```python
from build123d import *

# Parameters (mm, degrees)
SKETCH1_W                    = 91
SKETCH1_H                    = 32
BASE_FLANGE1_DEPTH           = 2
EDGE_FLANGE1_STRIP_W         = 14
EDGE_FLANGE1_STRIP_H         = 2
EDGE_FLANGE1_STRIP_CUT_DEPTH = 32
EDGE_FLANGE1_DEPTH           = 32
EDGE_FLANGE2_STRIP_W         = 14
EDGE_FLANGE2_STRIP_H         = 2
EDGE_FLANGE2_STRIP_CUT_DEPTH = 32
EDGE_FLANGE2_DEPTH           = 32
FILLET1_R                    = 3
EDGE_FLANGE3_DEPTH           = 29
EDGE_FLANGE3_START           = 2
EDGE_FLANGE3_FLAT_DEPTH      = 2
EDGE_FLANGE4_DEPTH           = 20
EDGE_FLANGE4_START           = 2
EDGE_FLANGE4_PROFILE_R       = 4
EDGE_FLANGE4_FLAT_DEPTH      = 2
SKETCH18_R                   = 6.5
CUT_EXTRUDE1_DEPTH           = 10
EDGE_FLANGE5_DEPTH           = 6
EDGE_FLANGE5_START           = 2
EDGE_FLANGE5_FLAT_DEPTH      = 2
EDGE_FLANGE6_STRIP_W         = 14
EDGE_FLANGE6_STRIP_H         = 2
EDGE_FLANGE6_STRIP_CUT_DEPTH = 32
EDGE_FLANGE6_DEPTH           = 32
EDGE_FLANGE7_STRIP_W         = 14
EDGE_FLANGE7_STRIP_H         = 2
EDGE_FLANGE7_STRIP_CUT_DEPTH = 32
EDGE_FLANGE7_DEPTH           = 32
EDGE_FLANGE7_FLAT_DEPTH      = 2
CUT_EXTRUDE2_DEPTH           = 10


# Sheet-metal steps are written as plain solids
with BuildPart() as part:
    # Sketch1 → Base-Flange1 (new body)
    with BuildSketch(Plane(origin=(0, 0, 0), x_dir=(0, 1, 0), z_dir=(0, 0, 1))):
        with Locations((-3.5, -1)):
            Rectangle(SKETCH1_W, SKETCH1_H)
    extrude(amount=BASE_FLANGE1_DEPTH)

    # Edge-Flange1 strip (across the edge) → Edge-Flange1 strip cut (cut)
    with BuildSketch(Plane(origin=(-15, -49, 2), x_dir=(0, 1, 0), z_dir=(1, 0, 0))):
        with Locations((-2, -1)):
            Rectangle(EDGE_FLANGE1_STRIP_W, EDGE_FLANGE1_STRIP_H)
    extrude(amount=EDGE_FLANGE1_STRIP_CUT_DEPTH, mode=Mode.SUBTRACT)

    # Edge-Flange1 section (across the edge) → Edge-Flange1 (add)
    with BuildSketch(Plane(origin=(-15, -49, 2), x_dir=(0, 1, 0), z_dir=(1, 0, 0))):
        with BuildLine():
            Line((0, 3), (0, 41))
            Line((0, 41), (2, 41))
            Line((2, 41), (2, 3))
            ThreePointArc((2, 3), (2.878679656, 0.878679656), (5, 0))
            Line((5, 0), (5, -2))
            ThreePointArc((5, -2), (1.464466094, -0.535533906), (0, 3))
        make_face()
    extrude(amount=EDGE_FLANGE1_DEPTH)

    # Edge-Flange2 strip (across the edge) → Edge-Flange2 strip cut (cut)
    with BuildSketch(Plane(origin=(17, -49, 43), x_dir=(0, 0, -1), z_dir=(-1, 0, 0))):
        with Locations((-2, -1)):
            Rectangle(EDGE_FLANGE2_STRIP_W, EDGE_FLANGE2_STRIP_H)
    extrude(amount=EDGE_FLANGE2_STRIP_CUT_DEPTH, mode=Mode.SUBTRACT)

    # Edge-Flange2 section (across the edge) → Edge-Flange2 (add)
    with BuildSketch(Plane(origin=(17, -49, 43), x_dir=(0, 0, -1), z_dir=(-1, 0, 0))):
        with BuildLine():
            Line((0, 3), (0, 19))
            Line((0, 19), (2, 19))
            Line((2, 19), (2, 3))
            ThreePointArc((2, 3), (2.878679656, 0.878679656), (5, 0))
            Line((5, 0), (5, -2))
            ThreePointArc((5, -2), (1.464466094, -0.535533906), (0, 3))
        make_face()
    extrude(amount=EDGE_FLANGE2_DEPTH)

    # Fillet1
    fillet1_edges = [part.edges().sort_by_distance(p)[0] for p in [
        (17, -68, 42),
        (-15, -68, 42),
    ]]
    fillet(fillet1_edges, radius=FILLET1_R)

    # Edge-Flange3 bend section (across the edge) → Edge-Flange3 (add)
    with BuildSketch(Plane(origin=(20, -33, 2), x_dir=(-1, 0, 0), z_dir=(0, 1, 0))):
        with BuildLine():
            Line((-2, 3), (0, 3))
            ThreePointArc((0, 3), (0.878679656, 0.878679656), (3, 0))
            Line((3, 0), (3, -2))
            ThreePointArc((3, -2), (-0.535533906, -0.535533906), (-2, 3))
        make_face()
    extrude(amount=EDGE_FLANGE3_DEPTH)

    # Edge-Flange3 profile (on flange) → Edge-Flange3 flat (add)
    with BuildSketch(Plane(origin=(20, 0, 2), x_dir=(0, 1, 0), z_dir=(1, 0, 0)).offset(EDGE_FLANGE3_START)):
        with BuildLine():
            Line((-33, 41), (-33, 3))
            Line((-33, 3), (-4, 3))
            Line((-4, 3), (-4, 7))
            Line((-4, 7), (7.090242207, 7))
            ThreePointArc((7.090242207, 7), (9, 8.406009114), (8.22462093, 10.647174828))
            Line((8.22462093, 10.647174828), (-1, 17))
            Line((-1, 17), (-13, 17))
            Line((-13, 17), (-13, 41))
            Line((-13, 41), (-33, 41))
        make_face()
    extrude(amount=-EDGE_FLANGE3_FLAT_DEPTH)

    # Edge-Flange4 bend section (across the edge) → Edge-Flange4 (add)
    with BuildSketch(Plane(origin=(20, -33, 46), x_dir=(0, 0, -1), z_dir=(0, 1, 0))):
        with BuildLine():
            Line((-2, 3), (0, 3))
            ThreePointArc((0, 3), (0.878679656, 0.878679656), (3, 0))
            Line((3, 0), (3, -2))
            ThreePointArc((3, -2), (-0.535533906, -0.535533906), (-2, 3))
        make_face()
    extrude(amount=EDGE_FLANGE4_DEPTH)

    # Edge-Flange4 profile (on flange) → Edge-Flange4 flat (add)
    with BuildSketch(Plane(origin=(20, 0, 46), x_dir=(0, 1, 0), z_dir=(0, 0, 1)).offset(EDGE_FLANGE4_START)):
        with BuildLine():
            ThreePointArc((-13, 25), (-13.878679656, 27.121320344), (-16, 28))
            Line((-16, 28), (-30, 28))
            ThreePointArc((-30, 28), (-32.121320344, 27.121320344), (-33, 25))
            Line((-33, 25), (-33, 3))
            Line((-33, 3), (-13, 3))
            Line((-13, 3), (-13, 25))
        make_face()
        with Locations((-23, 20)):
            Circle(EDGE_FLANGE4_PROFILE_R, mode=Mode.SUBTRACT)
    extrude(amount=-EDGE_FLANGE4_FLAT_DEPTH)

    # Sketch18 → Cut-Extrude1 (cut)
    with BuildSketch(Plane.XY.offset(2)):
        with Locations((0, 2)):
            Circle(SKETCH18_R)
        with BuildLine():
            Line((17, -4), (14, -4))
            ThreePointArc((14, -4), (12.585786438, -3.414213562), (12, -2))
            Line((12, -2), (12, 15))
            ThreePointArc((12, 15), (12.585786438, 16.414213562), (14, 17))
            Line((14, 17), (17, 17))
            Line((17, 17), (17, -4))
        make_face()
    extrude(amount=-CUT_EXTRUDE1_DEPTH, mode=Mode.SUBTRACT)

    # Edge-Flange5 bend section (across the edge) → Edge-Flange5 (add)
    with BuildSketch(Plane(origin=(20, 17, 2), x_dir=(-1, 0, 0), z_dir=(0, 1, 0))):
        with BuildLine():
            Line((-2, 3), (0, 3))
            ThreePointArc((0, 3), (0.878679656, 0.878679656), (3, 0))
            Line((3, 0), (3, -2))
            ThreePointArc((3, -2), (-0.535533906, -0.535533906), (-2, 3))
        make_face()
    extrude(amount=EDGE_FLANGE5_DEPTH)

    # Edge-Flange5 profile (on flange) → Edge-Flange5 flat (add)
    with BuildSketch(Plane(origin=(20, 0, 2), x_dir=(0, 1, 0), z_dir=(1, 0, 0)).offset(EDGE_FLANGE5_START)):
        with BuildLine():
            Line((17, 3), (23, 3))
            Line((23, 3), (23, 15))
            ThreePointArc((23, 15), (22.414213562, 16.414213562), (21, 17))
            Line((21, 17), (19, 17))
            ThreePointArc((19, 17), (17.585786438, 16.414213562), (17, 15))
            Line((17, 15), (17, 3))
        make_face()
    extrude(amount=-EDGE_FLANGE5_FLAT_DEPTH)

    # Edge-Flange6 strip (across the edge) → Edge-Flange6 strip cut (cut)
    with BuildSketch(Plane(origin=(17, 42, 2), x_dir=(0, -1, 0), z_dir=(-1, 0, 0))):
        with Locations((-2, -1)):
            Rectangle(EDGE_FLANGE6_STRIP_W, EDGE_FLANGE6_STRIP_H)
    extrude(amount=EDGE_FLANGE6_STRIP_CUT_DEPTH, mode=Mode.SUBTRACT)

    # Edge-Flange6 section (across the edge) → Edge-Flange6 (add)
    with BuildSketch(Plane(origin=(17, 42, 2), x_dir=(0, -1, 0), z_dir=(-1, 0, 0))):
        with BuildLine():
            Line((0, 3), (0, 41))
            Line((0, 41), (2, 41))
            Line((2, 41), (2, 3))
            ThreePointArc((2, 3), (2.878679656, 0.878679656), (5, 0))
            Line((5, 0), (5, -2))
            ThreePointArc((5, -2), (1.464466094, -0.535533906), (0, 3))
        make_face()
    extrude(amount=EDGE_FLANGE6_DEPTH)

    # Edge-Flange7 strip (across the edge) → Edge-Flange7 strip cut (cut)
    with BuildSketch(Plane(origin=(-15, 42, 43), x_dir=(0, 0, -1), z_dir=(1, 0, 0))):
        with Locations((-2, -1)):
            Rectangle(EDGE_FLANGE7_STRIP_W, EDGE_FLANGE7_STRIP_H)
    extrude(amount=EDGE_FLANGE7_STRIP_CUT_DEPTH, mode=Mode.SUBTRACT)

    # Edge-Flange7 bend section (across the edge) → Edge-Flange7 (add)
    with BuildSketch(Plane(origin=(-15, 42, 43), x_dir=(0, 0, -1), z_dir=(1, 0, 0))):
        with BuildLine():
            Line((0, 3), (2, 3))
            ThreePointArc((2, 3), (2.878679656, 0.878679656), (5, 0))
            Line((5, 0), (5, -2))
            ThreePointArc((5, -2), (1.464466094, -0.535533906), (0, 3))
        make_face()
    extrude(amount=EDGE_FLANGE7_DEPTH)

    # Edge-Flange7 profile (on flange) → Edge-Flange7 flat (add)
    with BuildSketch(Plane(origin=(0, 42, 43), x_dir=(1, 0, 0), z_dir=(0, 0, 1))):
        with BuildLine():
            ThreePointArc((-12, 23), (-14.121320344, 22.121320344), (-15, 20))
            Line((-15, 20), (-15, 3))
            Line((-15, 3), (17, 3))
            Line((17, 3), (17, 20))
            ThreePointArc((17, 20), (16.121320344, 22.121320344), (14, 23))
            Line((14, 23), (-12, 23))
        make_face()
        with BuildLine():
            Line((-5, 17.5), (5, 17.5))
            ThreePointArc((5, 17.5), (7.5, 15), (5, 12.5))
            Line((5, 12.5), (-5, 12.5))
            ThreePointArc((-5, 12.5), (-7.5, 15), (-5, 17.5))
        make_face(mode=Mode.SUBTRACT)
    extrude(amount=-EDGE_FLANGE7_FLAT_DEPTH)

    # Sketch28 → Cut-Extrude2 (cut)
    with BuildSketch(Plane.XY.offset(43)):
        with BuildLine():
            Line((-5, -57.5), (5, -57.5))
            ThreePointArc((5, -57.5), (7.5, -60), (5, -62.5))
            Line((5, -62.5), (-5, -62.5))
            ThreePointArc((-5, -62.5), (-7.5, -60), (-5, -57.5))
        make_face()
    extrude(amount=-CUT_EXTRUDE2_DEPTH, mode=Mode.SUBTRACT)


solid = part.part
```
Verification items for the finished model (mm, model axes). A direction names the side the tool comes from. Coordinates: 2 decimals unless noted, no trailing zeros. Loops run counter-clockwise (first coordinate to the right, second up) from the corner with the lowest first, then second, coordinate; pieces in that order, holes last. Notation, with made-up numbers: (89, -35.5) -> (104, -35.5) arc R14 cw to (104, -10.5) -> close; hole circle Ø8 at (17, 52). An arc over 180 degrees is marked (long way). Answer in a Markdown table with one row per item.
1) Access from +Z, -Z, +X, -X, +Y, -Y to the whole of each face (thin tool, end or side, straight path). Record for faces 4 (the face through (1.22, 39.14, 2.9)), 5 (the face through (-3, -4, 2)), 6 (the face through (1, -49, 21)), 7 (the face through (4.3, -23.1, 46)), 8 (the face through (17, 41, 22)).
The answers:
| item | result |
|---|---|
| face 4 | +Z, +X, -X |
| face 5 | -X |
| face 6 | -Z, +X, -X, -Y |
| face 7 | -X, +Y, -Y |
| face 8 | +Z, -Z, +X, +Y |
2) Section check D-D (x = 0). Give the number of separate pieces and of enclosed holes in the cut face, and give its area (3 significant figures).
The answers:
| item | result |
|---|---|
| separate pieces | 6 |
| enclosed holes | 0 |
| area | 394 mm2 |
3) Section check B-B (z = 33). Record the cut outline in (x, y).
The answers:
| item | result |
|---|---|
| outline | (-15, -49) -> (17, -49) -> (17, -47) -> (-15, -47) -> close; (-15, 40) -> (17, 40) -> (17, 42) -> (-15, 42) -> close; (20, -33) -> (22, -33) -> (22, -13) -> (20, -13) -> close |
4) Section check A-A (y = -23). Record the cut outline in (x, z).
The answers:
| item | result |
|---|---|
| outline | (-15, 0) -> (17, 0) arc R5 ccw to (22, 5) -> (22, 43) arc R5 ccw to (17, 48) -> (4, 48) -> (4, 46) -> (17, 46) arc R3 cw to (20, 43) -> (20, 5) arc R3 cw to (17, 2) -> (-15, 2) -> close; (-8, 46) -> (-4, 46) -> (-4, 48) -> (-8, 48) -> close |
5) Depth check by flat-ended pin: P1, Ø19, axis at y = -15, z = 25, coming from the -X side; P2, Ø16, axis at x = -1.5, z = 20.5, coming from the -Y side; P3, Ø11.5, axis at y = 41.5, z = 19, coming from the +X side; P4, Ø6, axis at y = -8, z = 41.5, coming from the +X side (1 decimal). Enter the tip coordinate at first touch or a pass-through.
The answers:
| item | result |
|---|---|
| P1 | stops at x = 20 |
| P2 | stops at y = -49 |
| P3 | stops at x = 17 |
| P4 | passes through |
6) Section check C-C (x = 10.5). Record the cut outline in (y, z), and give its area (3 significant figures).
The answers:
| item | result |
|---|---|
| outline | (-68, 41) -> (-52, 41) arc R3 cw to (-49, 38) -> (-49, 5) arc R5 ccw to (-44, 0) -> (37, 0) arc R5 ccw to (42, 5) -> (42, 38) arc R3 cw to (45, 41) -> (65, 41) -> (65, 43) -> (45, 43) arc R5 ccw to (40, 38) -> (40, 5) arc R3 cw to (37, 2) -> (-44, 2) arc R3 cw to (-47, 5) -> (-47, 38) arc R5 ccw to (-52, 43) -> (-68, 43) -> close; (-33, 46) -> (-13, 46) -> (-13, 48) -> (-33, 48) -> close |
| area | 456 mm2 |
7) Scan lines: line 1 along Y through (x, z) = (0, 29); line 2 along Y through (x, z) = (0, 47.45); line 3 along Z through (x, y) = (-8.5, 36.5). Record each from-to range of solid material in increasing order. Write a range as from..to.
The answers:
| item | result |
|---|---|
| line 1 | y = -49..-47, 40..42 |
| line 2 | y = -33..-27, -19..-13 |
| line 3 | z = 0..2 |
8) Draft check along X on faces 1 (the face through (1, -47, 1)), 2 (the face through (-7.5, 56.9, 42)), 3 (the face through (22, 20, 12)). Enter one of: released by +X, released by -X, zero draft, split by the parting line, or undercut.
The answers:
| item | result |
|---|---|
| face 1 | zero draft |
| face 2 | undercut |
| face 3 | released by +X |
